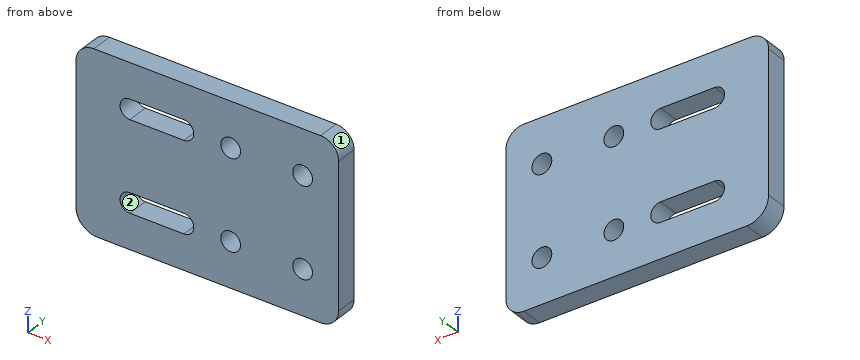
Autodesk Inventor part; units mm, degrees
ref_plane "YZ Plane" through (0, 0, 0) normal (1, 0, 0) x (0, 1, 0)
ref_plane "XZ Plane" through (0, 0, 0) normal (0, 1, 0) x (-1, 0, 0)
ref_plane "XY Plane" through (0, 0, 0) normal (0, 0, 1) x (1, 0, 0)
sketch "Sketch1" plane through (0, 0, 0) normal (0, 1, 0) x (-1, 0, 0)
  line L0 (0, 0) -> (105, 0)
  line L1 (105, 0) -> (105, -50)
  line L2 (105, -50) -> (0, -50)
  line L3 (0, -50) -> (0, 0)
  line L4 (0, 0) -> (0, -16.6667)
  line L5 (0, -16.6667) -> (11, -16.6667)
  dimension "d0" = 105
  dimension "d1" = 50
  dimension "d2" = 16.6667
  dimension "d3" = 11
extrude "Extrusion1" add sketch "Sketch1" along normal blind 6
sketch "Sketch3" plane through (0, 6, 0) normal (0, 1, 0) x (1, 0, 0)
  circle A0 centre (-20, 12.5) radius 2.75
  line L0 (0, 0) -> (0, 50)
  line L1 (-105, 0) -> (0, 0)
  circle A1 centre (-20, 37.5) radius 2.75
  dimension "d21" = 5.5
  dimension "d22" = 20
  dimension "d23" = 12.5
  dimension "d26" = 25
extrude "Extrusion3" cut sketch "Sketch3" against normal through all
sketch "Sketch4" plane through (0, 6, 0) normal (0, 1, 0) x (1, 0, 0)
  circle A0 centre (-20, 12.5) radius 2.75
  line L0 (-20, 12.5) -> (-75, 12.5)
  line L1 (-75, 12.5) -> (-90, 12.5) construction
  line L2 (-75, 15.25) -> (-90, 15.25)
  line L3 (-90, 9.75) -> (-75, 9.75)
  arc A1 (-75, 9.75) -> (-75, 15.25) centre (-75, 12.5) ccw
  arc A2 (-90, 15.25) -> (-90, 9.75) centre (-90, 12.5) ccw
  point P0 (0, 0)
  point P1 (-82.5, 12.5)
  dimension "d33" = 55
  dimension "d34" = 15
  dimension "d35" = 5.5
extrude "Extrusion4" cut sketch "Sketch4" against normal through all contours A1 L3 A2 L2
pattern_linear "Rectangular Pattern2" count 2 spacing 25 along (0, 0, -1) of "Extrusion4"
fillet "Fillet2" radius 5 3 edges at (-105, 3, 0) (0, 3, 0) (0, 3, -50)
sketch "Sketch7" plane through (0, 6, 0) normal (0, 1, 0) x (1, 0, 0)
  circle A0 centre (-20, 12.5) radius 2.75
  line L0 (-20, 12.5) -> (-42, 12.5)
  line L1 (-42, 12.5) -> (-62, 12.5)
  circle A1 centre (-62, 12.5) radius 2.75
  circle A2 centre (-42, 12.5) radius 2.75
  line L2 (0, 5) -> (0, 45)
  line L3 (0, 0) -> (0, 45)
  circle A3 centre (-42, 37.5) radius 2.75
  circle A4 centre (-62, 37.5) radius 2.75
  dimension "d55" = 22
  dimension "d56" = 20
  dimension "d57" = 5.5
  dimension "d58" = 5.5
  dimension "d61" = 25
extrude "Extrusion7" cut sketch "Sketch7" against normal through all contours A2 L1 L0 | L0 L1 A2 | A1 | A3 | A4
sketch "Sketch9" plane through (0, 6, 0) normal (0, 1, 0) x (1, 0, 0)
  point P0 (0, 0)
sketch "Sketch12" plane through (0, 6, 0) normal (0, 1, 0) x (1, 0, 0)
  circle A0 centre (-42, 37.5) radius 2.75
  line L0 (-42, 37.5) -> (-32, 37.5)
  line L1 (-32, 37.5) -> (-32, 50)
  line L2 (-5, 50) -> (-105, 50)
  line L3 (-32, 50) -> (0, 50)
  line L4 (0, 50) -> (0, 0)
  line L5 (0, 0) -> (-32, 0)
  line L6 (-32, 0) -> (-32, 50)
  point P0 (-74, 50)
  dimension "d87" = 10
extrude "Extrusion10" cut sketch "Sketch12" against normal blind 10 contours L1 L2 L3 L4 L5 L6
fillet "Fillet3" radius 5 2 edges at (-32, 3, 0) (-32, 3, -50)
fillet "Fillet4" radius 6 1 edges at (-105, 3, -50)
properties part number "X_Carriage_Plate_Short"
Geometry check sheet. Reference: the model listing, model coordinates, mm. Face numbers are marked on the shaded views. A direction names the side the tool comes from. Coordinates: 2 decimals unless noted, no trailing zeros. Write each loop counter-clockwise with the first axis right and the second up, starting at its lowest first coordinate (ties: lowest second). Pieces come first, ordered by that corner, then holes. Notation, with made-up numbers: M 26.5,-10.75 L 35.5,-10.75 A15 cw 35.5,6.25 Z; hole C 57.25,-10 d6. An arc over 180 degrees is marked long. Answer as a JSON object with one key per item and string values.
1. Section check B-B, the plane y = 4.6. Enter the section's corners in (x, z).
Answers below:
{"outline": "M -105,-44 A6 ccw -99,-50 L -37,-50 A5 ccw -32,-45 L -32,-5 A5 ccw -37,0 L -100,0 A5 ccw -105,-5 Z; hole M -90,-40.25 L -75,-40.25 A2.75 ccw -75,-34.75 L -90,-34.75 A2.75 ccw Z; hole M -90,-15.25 L -75,-15.25 A2.75 ccw -75,-9.75 L -90,-9.75 A2.75 ccw Z; hole C -62,-37.5 d5.5; hole C -62,-12.5 d5.5; hole C -42,-37.5 d5.5; hole C -42,-12.5 d5.5"}
2. Scan lines: L1, parallel to X at y = 2.9, z = -12.5; L2, parallel to Z at x = -42, y = 1.7; L3, parallel to Z at x = -41, y = 1.7. Record each from-to range of solid material in increasing order.
Answers below:
{"L1": "x = -105 to -92.75, -72.25 to -64.75, -59.25 to -44.75, -39.25 to -32", "L2": "z = -50 to -40.25, -34.75 to -15.25, -9.75 to 0", "L3": "z = -50 to -40.06, -34.94 to -15.06, -9.94 to 0"}
3. Section check A-A, the plane z = -37.5. Enter the section's corners in (x, y).
Answers below:
{"outline": "M -105,0 L -92.75,0 L -92.75,6 L -105,6 Z; M -72.25,0 L -64.75,0 L -64.75,6 L -72.25,6 Z; M -59.25,0 L -44.75,0 L -44.75,6 L -59.25,6 Z; M -39.25,0 L -32,0 L -32,6 L -39.25,6 Z"}
4. Tool access check on the marked faces 1 and 2. Record the directions out of +Z, -Z, +X, -X, +Y, -Y that give a thin tool (end or side, any length) a straight path to the whole face; none if there is none.
Answers below:
{"face 1": "+Z, +X, +Y, -Y", "face 2": "+Y, -Y"}
5. Section check C-C, the plane x = -42. Enter the section's corners in (y, z), plus the area to 3 significant figures.
Answers below:
{"outline": "M 0,-50 L 6,-50 L 6,-40.25 L 0,-40.25 Z; M 0,-34.75 L 6,-34.75 L 6,-15.25 L 0,-15.25 Z; M 0,-9.75 L 6,-9.75 L 6,0 L 0,0 Z", "area": "234 mm²"}
